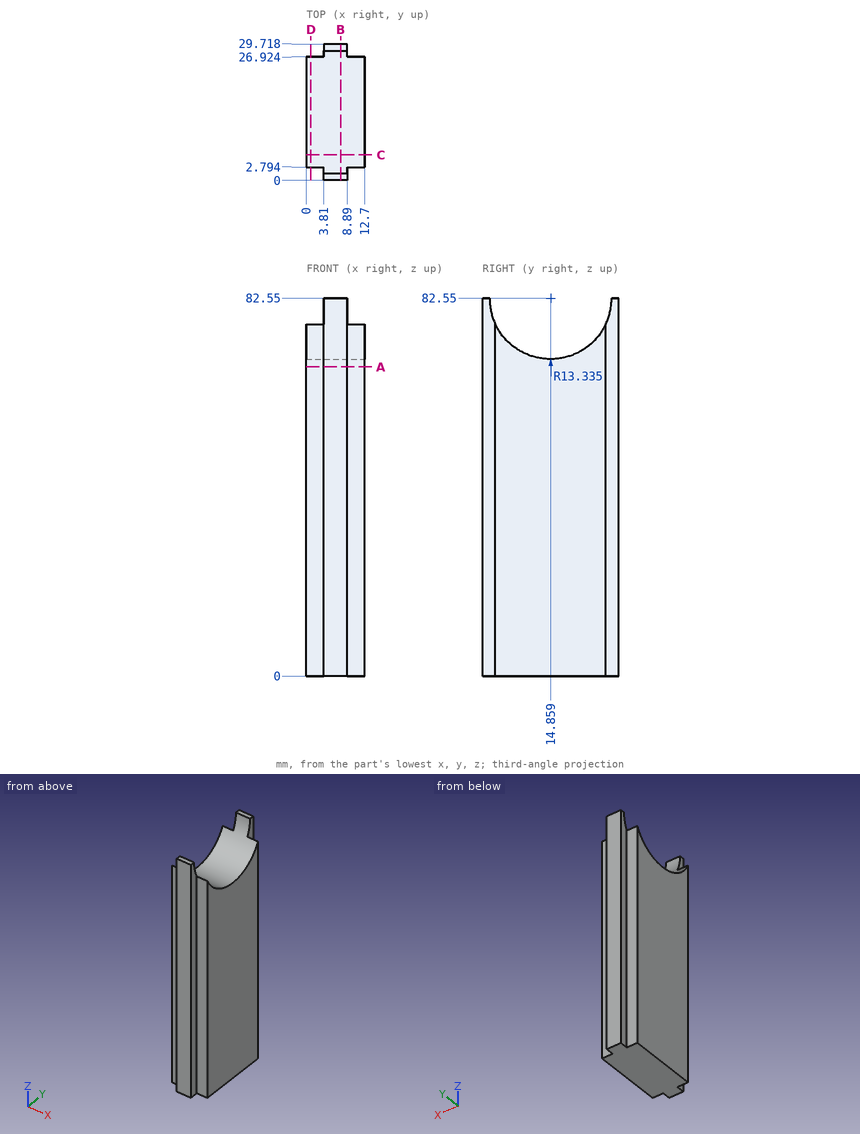
Here's the drawing with two shaded views (mm, measured from the low corner). I have some questions. Give positions to 0.01 mm unless a question says otherwise; leave off trailing zeros. Loops run counter-clockwise (first coordinate to the right, second up) from the corner with the lowest first, then second, coordinate; pieces in that order, holes last. Notation, with made-up numbers: (30.5, -6.5) - (64.5, -6.5) arc R34 ccw to (64.5, 23.5) - close; hole circle Ø10 at (66, 46.25). An arc over 180 degrees is marked (long way). One line per item, written item: value.
(1) If we section it at C-C, the plane y = 5.5: List the corners of the cut face in (x, z) for me, plus the area to 3 significant figures.
Verdict:
outline: (0, 0) - (12.7, 0) - (12.7, 73.05) - (0, 73.05) - close
area: 928 mm^2
(2) If we section it at D-D, the plane x = 1: List the corners of the cut face in (y, z) for me (3 decimals).
Verdict:
outline: (2.794, 0) - (26.924, 0) - (26.924, 76.87) arc R13.335 cw to (2.794, 76.87) - close
(3) If we section it at A-A, the plane z = 67.5: List the corners of the cut face in (x, y) for me.
Verdict:
outline: (0, 2.79) - (3.81, 2.79) - (3.81, 0) - (8.89, 0) - (8.89, 2.79) - (12.7, 2.79) - (12.7, 26.92) - (8.89, 26.92) - (8.89, 29.72) - (3.81, 29.72) - (3.81, 26.92) - (0, 26.92) - close
(4) I need wall thicknesses on line 1 along Y through (x, z) = (9.75, 49); line 2 along X through (y, z) = (27, 21.5); line 3 along Y through (x, z) = (1, 74.5). Which ranges of each line are inside material? Lowest first, please.
Verdict:
line 1: 2.79 to 26.92
line 2: 3.81 to 8.89
line 3: 2.79 to 4.23, 25.49 to 26.92
(5) If we section it at B-B, the plane x = 7.5: List the corners of the cut face in (y, z) for me (3 decimals), plus the area to 3 significant figures.
Verdict:
outline: (0, 0) - (29.718, 0) - (29.718, 82.55) - (28.194, 82.55) arc R13.335 cw to (1.524, 82.55) - (0, 82.55) - close
area: 2,170 mm^2
(6) I'm going to push flat-ended pins straight in: pin 1 (2 mm diameter, centred on y = 1, z = 21.5, fed in from +X); pin 2 (3 mm diameter, centred on y = 2, z = 50.5, fed in from -X); pin 3 (1.9 mm diameter, centred on x = 10, z = 29.5, fed in from -Y); pin 4 (3 mm diameter, centred on y = 29, z = 41.5, fed in from -X). Where does each tip first touch, or does it pass through?
Verdict:
pin 1: x = 8.89
pin 2: x = 0
pin 3: y = 2.79
pin 4: x = 3.81
